from build123d import *

# Parameters (mm, degrees)
SKETCH1_W           = 7.62
SKETCH1_H           = 5.8
BOSS_EXTRUDE1_DEPTH = 3.16
SKETCH2_W           = 5.08
SKETCH2_H           = 1
BOSS_EXTRUDE2_DEPTH = 8.54
SKETCH3_W           = 5.08
SKETCH3_H           = 6.25
BOSS_EXTRUDE3_DEPTH = 0.53
SKETCH4_W           = 1.68
SKETCH4_H           = 0.64
CUT_EXTRUDE1_DEPTH  = 13.270717175
SKETCH5_W           = 1.68
SKETCH5_H           = 0.64
CUT_EXTRUDE2_DEPTH  = 13.270717175
SKETCH6_W           = 0.53
SKETCH6_H           = 3.802013072
CUT_EXTRUDE3_DEPTH  = 13.298914586
SKETCH7_W           = 1.68
SKETCH7_H           = 0.64
CUT_EXTRUDE4_DEPTH  = 13.270717175
SKETCH8_W           = 0.64
SKETCH8_H           = 0.64
BOSS_EXTRUDE4_DEPTH = 4.2
SKETCH9_W           = 0.64
SKETCH9_H           = 0.64
BOSS_EXTRUDE5_DEPTH = 4.2
SKETCH10_W          = 0.64
SKETCH10_H          = 0.635
BOSS_EXTRUDE6_DEPTH = 4.2
SKETCH11_W          = 0.64
SKETCH11_H          = 0.64
BOSS_EXTRUDE7_DEPTH = 7.5
SKETCH12_W          = 0.64
SKETCH12_H          = 0.64
BOSS_EXTRUDE8_DEPTH = 7.5
SKETCH13_W          = 0.64
SKETCH13_H          = 0.64
BOSS_EXTRUDE9_DEPTH = 7.5
DRAFT1_ANGLE        = 45
DRAFT2_ANGLE        = 60
CHAMFER1_SIZE       = 0.75
CHAMFER1_SIZE2      = 0.272977676
CHAMFER2_SIZE       = 0.272977676
CHAMFER2_SIZE2      = 0.75
FILLET1_R           = 0.25


with BuildPart() as part:
    # Sketch1 → Boss-Extrude1 (new body)
    with BuildSketch(Plane.XZ.offset(1.58)):
        with Locations((0, 0.02)):
            Rectangle(SKETCH1_W, SKETCH1_H)
    extrude(amount=-BOSS_EXTRUDE1_DEPTH)

    # Sketch2 → Boss-Extrude2 (add)
    with BuildSketch(Plane(origin=(0, 1.58, 0), x_dir=(-1, 0, 0), z_dir=(0, 1, 0))):
        with Locations((0, -2.38)):
            Rectangle(SKETCH2_W, SKETCH2_H)
    extrude(amount=BOSS_EXTRUDE2_DEPTH)

    # Sketch3 → Boss-Extrude3 (add)
    with BuildSketch(Plane.XY.offset(-1.88)):
        with Locations((0, 6.995)):
            Rectangle(SKETCH3_W, SKETCH3_H)
    extrude(amount=BOSS_EXTRUDE3_DEPTH)

    # Sketch4 → Cut-Extrude1 (cut, through all)
    with BuildSketch(Plane(origin=(0, 0, -2.88), x_dir=(-1, 0, 0), z_dir=(0, 0, -1))):
        with Locations((2.54, -1.26)):
            Rectangle(SKETCH4_W, SKETCH4_H)
    extrude(amount=-CUT_EXTRUDE1_DEPTH, mode=Mode.SUBTRACT)

    # Sketch5 → Cut-Extrude2 (cut, through all)
    with BuildSketch(Plane(origin=(0, 0, -2.88), x_dir=(-1, 0, 0), z_dir=(0, 0, -1))):
        with Locations((0, -1.26)):
            Rectangle(SKETCH5_W, SKETCH5_H)
    extrude(amount=-CUT_EXTRUDE2_DEPTH, mode=Mode.SUBTRACT)

    # Sketch6 → Cut-Extrude3 (cut, through all)
    with BuildSketch(Plane(origin=(2.54, 0, 0), x_dir=(0, 0, -1), z_dir=(1, 0, 0))):
        with Locations((1.615, 8.218993464)):
            Rectangle(SKETCH6_W, SKETCH6_H)
    extrude(amount=-CUT_EXTRUDE3_DEPTH, mode=Mode.SUBTRACT)

    # Sketch7 → Cut-Extrude4 (cut, through all)
    with BuildSketch(Plane(origin=(0, 0, -2.88), x_dir=(-1, 0, 0), z_dir=(0, 0, -1))):
        with Locations((-2.54, -1.26)):
            Rectangle(SKETCH7_W, SKETCH7_H)
    extrude(amount=-CUT_EXTRUDE4_DEPTH, mode=Mode.SUBTRACT)

    # Sketch8 → Boss-Extrude4 (add)
    with BuildSketch(Plane.XZ.offset(0.94)):
        Rectangle(SKETCH8_W, SKETCH8_H)
    extrude(amount=BOSS_EXTRUDE4_DEPTH)

    # Sketch9 → Boss-Extrude5 (add)
    with BuildSketch(Plane.XZ.offset(0.94)):
        with Locations((-2.54, 0)):
            Rectangle(SKETCH9_W, SKETCH9_H)
    extrude(amount=BOSS_EXTRUDE5_DEPTH)

    # Sketch10 → Boss-Extrude6 (add)
    with BuildSketch(Plane.XZ.offset(0.94)):
        with Locations((2.54, 0.0025)):
            Rectangle(SKETCH10_W, SKETCH10_H)
    extrude(amount=BOSS_EXTRUDE6_DEPTH)

    # Sketch11 → Boss-Extrude7 (add)
    with BuildSketch(Plane(origin=(0, 1.58, 0), x_dir=(-1, 0, 0), z_dir=(0, 1, 0))):
        Rectangle(SKETCH11_W, SKETCH11_H)
    extrude(amount=BOSS_EXTRUDE7_DEPTH)

    # Sketch12 → Boss-Extrude8 (add)
    with BuildSketch(Plane(origin=(0, 1.58, 0), x_dir=(-1, 0, 0), z_dir=(0, 1, 0))):
        with Locations((-2.54, 0)):
            Rectangle(SKETCH12_W, SKETCH12_H)
    extrude(amount=BOSS_EXTRUDE8_DEPTH)

    # Sketch13 → Boss-Extrude9 (add)
    with BuildSketch(Plane(origin=(0, 1.58, 0), x_dir=(-1, 0, 0), z_dir=(0, 1, 0))):
        with Locations((2.54, 0)):
            Rectangle(SKETCH13_W, SKETCH13_H)
    extrude(amount=BOSS_EXTRUDE9_DEPTH)

    # Draft1
    draft1_faces = [part.faces().sort_by_distance(p)[0] for p in [
        (0, 3.87, -1.615),
    ]]
    draft(draft1_faces, Plane(origin=(2.54, 10.12, -1.88), x_dir=(1, 0, 0), z_dir=(0, 0, 1)), DRAFT1_ANGLE)

    # Draft2
    draft2_faces = [part.faces().sort_by_distance(p)[0] for p in [
        (0, 6.317986928, -1.615),
    ]]
    draft(draft2_faces, Plane(origin=(-3.810025, 6.317986928, -1.88), x_dir=(1, 0, 0), z_dir=(0, 0, 1)), DRAFT2_ANGLE)

    # Chamfer1
    chamfer1_edges = [part.edges().sort_by_distance(p)[0] for p in [
        (2.54, 10.12, -2.38),
    ]]
    chamfer1_side = [part.faces().sort_by_distance(p)[0] for p in [
        (2.54, 5.768868228, -2.309646908),
    ]]
    chamfer(chamfer1_edges, length=CHAMFER1_SIZE, length2=CHAMFER1_SIZE2, reference=chamfer1_side[0])

    # Chamfer2
    chamfer2_edges = [part.edges().sort_by_distance(p)[0] for p in [
        (-2.54, 10.12, -2.38),
    ]]
    chamfer2_side = [part.faces().sort_by_distance(p)[0] for p in [
        (-0.136488838, 10.12, -2.38),
    ]]
    chamfer(chamfer2_edges, length=CHAMFER2_SIZE, length2=CHAMFER2_SIZE2, reference=chamfer2_side[0])

    # Fillet1
    fillet1_edges = [part.edges().sort_by_distance(p)[0] for p in [
        (0, 1.58, -1.88),
    ]]
    fillet(fillet1_edges, radius=FILLET1_R)


solid = part.part
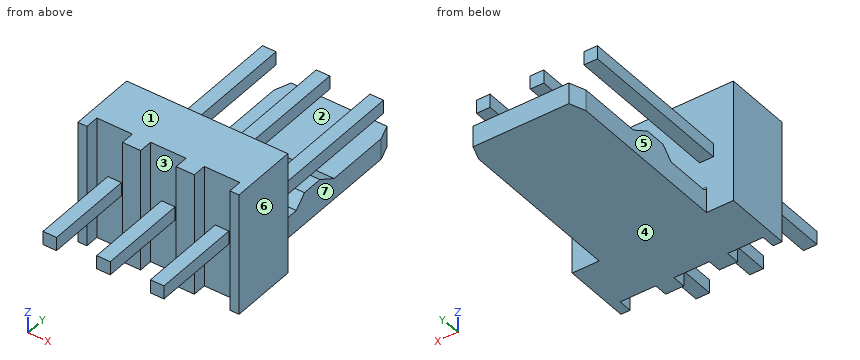
Part model, mm, in its own coordinate system. Face numbers are marked on the shaded views. A direction names the side the tool comes from. Coordinates: 2 decimals unless noted, no trailing zeros. Loops run counter-clockwise (first coordinate to the right, second up) from the corner with the lowest first, then second, coordinate; pieces in that order, holes last. Notation, with made-up numbers: (15.5, 48) - (73.5, 48) arc R28 ccw to (73.5, 72) - close; hole circle Ø10 at (-9.5, 41.25). An arc over 180 degrees is marked (long way). Write each question's results on one line, items separated by ' | '. Start each with the question number.
Q1. Which spindle directions (+Z, -Z, +X, -X, +Y, -Y) get a long thin tool onto all of the face, cutting with end or side? Do the marked faces 5, 6 and 7. Say none if no direction does.
Q2. Drop flat-ended pins along their axis: pin 1 Ø3 at (y, z) = (-2.5, 0) entering from -X; pin 2 Ø0.7 at (x, z) = (0, 0) entering from +Y; pin 3 Ø0.5 at (x, z) = (-3.5, 1) entering from -Y; pin 4 Ø0.8 at (x, y) = (-0.5, 5) entering from +Z. Give the stop position or say it passes through.
Q3. Probe line 1 along X through (y, z) = (-1.5, -0.8); line 2 along Z through (x, y) = (0.25, 7); line 3 along X through (y, z) = (7.75, -2.05). List the from-to ranges inside material, lowest first.
Q4. Two-plate mould, pull along Z, no slides. Class the marked faces 1, 2, 3 and 4: +Z half, -Z half, draft (parallel to the pull), parting line (faces both ways), or undercut.
Q5. Slice it at A-A on y = 7.75. Give the cut face in (x, z), and give its area (3 significant figures).
Q6. Slice it at C-C on z = -0.6. Give the cut face in (x, y), and give its area (3 significant figures).
Q7. Slice it at B-B on x = 2. Give the cut face in (y, z).
Answer:
1) face 5: -Z, -X, +Y | face 6: +Z, -Z, +X, +Y, -Y | face 7: -Z, +X, +Y
2) pin 1: stops at x = -3.81 | pin 2: stops at y = 9.08 | pin 3: stops at y = -1.58 | pin 4: stops at z = 0.32
3) line 1: x = -3.81 to -3.38, -1.7 to -0.84, 0.84 to 1.7, 3.38 to 3.81 | line 2: z = -2.88 to -1.88, -0.32 to 0.32 | line 3: x = -2.54 to 2.54
4) face 1: +Z half | face 2: undercut | face 3: draft | face 4: -Z half
5) outline: (-2.86, -0.32) - (-2.22, -0.32) - (-2.22, 0.32) - (-2.86, 0.32) - close; (-2.54, -2.88) - (2.54, -2.88) - (2.54, -1.88) - (-2.54, -1.88) - close; (-0.32, -0.32) - (0.32, -0.32) - (0.32, 0.32) - (-0.32, 0.32) - close; (2.22, -0.32) - (2.86, -0.32) - (2.86, 0.32) - (2.22, 0.32) - close | area: 6.31 mm2
6) outline: (-3.81, -1.58) - (-3.38, -1.58) - (-3.38, -0.94) - (-1.7, -0.94) - (-1.7, -1.58) - (-0.84, -1.58) - (-0.84, -0.94) - (0.84, -0.94) - (0.84, -1.58) - (1.7, -1.58) - (1.7, -0.94) - (3.38, -0.94) - (3.38, -1.58) - (3.81, -1.58) - (3.81, 1.58) - (-3.81, 1.58) - close | area: 20.9 mm2
7) outline: (-0.94, -2.88) - (10.12, -2.88) - (10.12, -1.88) - (6.32, -1.88) - (5.4, -1.35) - (4.4, -1.35) - (3.87, -1.88) - (1.83, -1.88) arc R0.25 cw to (1.58, -1.63) - (1.58, 2.92) - (-0.94, 2.92) - close
